Input: part model. Units: mm. Frame: model coordinates. Face numbers are marked on the shaded views. A direction names the side the tool comes from. Coordinates: 2 decimals unless noted, no trailing zeros. Order: outer loops, then holes, each group sorted by start corner. A loop starts at its lowest first (then second) coordinate and runs counter-clockwise, first axis right, second up. Notation, with made-up numbers: (88.25, 11) -> (101.25, 11) arc R28 ccw to (101.25, 33) -> close; hole circle Ø5 at (52.25, 34.25). An arc over 180 degrees is marked (long way). Write each question's results on one line, items separated by ' | '.
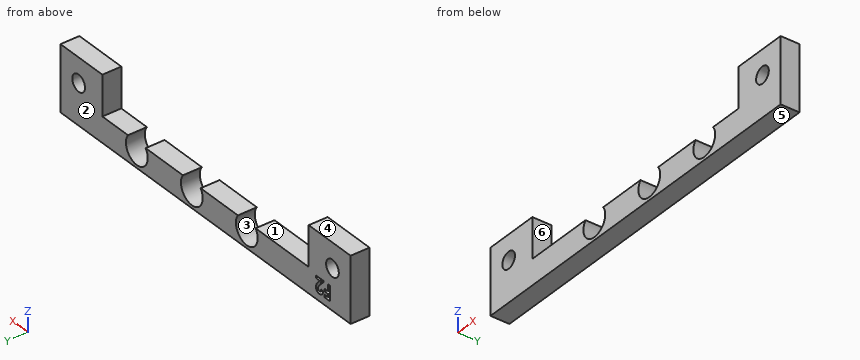
```python
from build123d import *

# Parameters (mm, degrees)
BOSS_EXTRUDE1_OUTLINE_R = 1.75
BOSS_EXTRUDE1_DEPTH     = 4
CUT_EXTRUDE1_DEPTH      = 1


# Read off the part's stored shape, not the designer's step: Boss-Extrude1
with BuildPart() as part:
    # Boss-Extrude1 outline → Boss-Extrude1 (new body)
    with BuildSketch(Plane(origin=(0, 0, 0), x_dir=(1, 0, 0), z_dir=(0, 1, 0))):
        with BuildLine():
            Line((59.039776182, -18.816315938), (59.039776182, -4.977921029))
            Line((59.039776182, -4.977921029), (-20.960223818, -4.977921029))
            Line((-20.960223818, -4.977921029), (-20.960223818, -18.816315938))
            Line((-20.960223818, -18.816315938), (-9.410223818, -18.816315938))
            Line((-9.410223818, -18.816315938), (-9.410223818, -10.337441858))
            Line((-9.410223818, -10.337441858), (5.23307726, -10.337441858))
            ThreePointArc((5.23307726, -10.337441858), (7.669776182, -5.587442326), (10.106475105, -10.337441858))
            Line((10.106475105, -10.337441858), (20.39307726, -10.337441858))
            ThreePointArc((20.39307726, -10.337441858), (22.829776183, -5.587442326), (25.266475105, -10.337441858))
            Line((25.266475105, -10.337441858), (35.55307726, -10.337441858))
            ThreePointArc((35.55307726, -10.337441858), (37.989776182, -5.587442326), (40.426475105, -10.337441858))
            Line((40.426475105, -10.337441858), (47.489776182, -10.337441858))
            Line((47.489776182, -10.337441858), (47.489776182, -18.816315938))
            Line((47.489776182, -18.816315938), (59.039776182, -18.816315938))
        make_face()
        with Locations((-15.960223818, -13.587442209)):
            Circle(BOSS_EXTRUDE1_OUTLINE_R, mode=Mode.SUBTRACT)
        with Locations((54.039776182, -13.587442209)):
            Circle(BOSS_EXTRUDE1_OUTLINE_R, mode=Mode.SUBTRACT)
    extrude(amount=BOSS_EXTRUDE1_DEPTH)

    # Sketch2 → Cut-Extrude1 (cut)
    with BuildSketch(Plane(origin=(0, 4, 0), x_dir=(1, 0, 0), z_dir=(0, 1, 0))):
        Polygon((-15.320752279, -6.539659084), (-13.773957408, -6.539659084), (-13.773957408, -7.109530878), (-14.750880484, -7.109530878), (-14.750880484, -7.720107802), (-13.773957408, -7.720107802), (-13.773957408, -8.289979596), (-14.750880484, -8.289979596), (-14.750880484, -9.714659084), (-15.320752279, -9.714659084), align=None)
        with BuildLine():
            Line((-12.837739459, -7.597992417), (-13.407611254, -7.597992417))
            add(Edge.make_bspline(
                [(-13.407611254, -7.597992417), (-13.405150065, -7.554884631), (-13.40034105, -7.470654604), (-13.381212002, -7.348307794), (-13.355579735, -7.232703511), (-13.321370072, -7.124246154), (-13.278383392, -7.022975131), (-13.227725853, -6.928545205), (-13.16810327, -6.84145355), (-13.100784607, -6.762120173), (-13.026912751, -6.690949467), (-12.948021354, -6.627845049), (-12.862903665, -6.575772871), (-12.773114854, -6.53292229), (-12.678670211, -6.498686666), (-12.57867614, -6.475797382), (-12.473998445, -6.460296534), (-12.402338086, -6.458940148), (-12.365814379, -6.458248827)],
                knots=[0, 0, 0, 0, 1.199038563, 2.342849363, 3.436047546, 4.486744587, 5.497670872, 6.488682221, 7.459191391, 8.424610317, 9.374430501, 10.305433194, 11.225809216, 12.140057399, 13.06607119, 14.010487599, 14.985989317, 16, 16, 16, 16], degree=3))
            add(Edge.make_bspline(
                [(-12.365814379, -6.458248827), (-12.320982046, -6.459647714), (-12.233458825, -6.462378669), (-12.106280643, -6.485674624), (-11.987510127, -6.524640707), (-11.877233611, -6.579086602), (-11.776389898, -6.648254404), (-11.684995712, -6.730725688), (-11.605814958, -6.828230745), (-11.538345606, -6.936712548), (-11.482286639, -7.05157951), (-11.44300285, -7.170356712), (-11.417182038, -7.289892289), (-11.414428089, -7.370381495), (-11.413059972, -7.410367217)],
                knots=[0, 0, 0, 0, 1.075374347, 2.099382735, 3.09057751, 4.06680945, 5.040638231, 6.016817125, 7.011024321, 8.044445721, 9.0776792, 10.070479129, 11.0414456, 12, 12, 12, 12], degree=3))
            add(Edge.make_bspline(
                [(-11.413059972, -7.410367217), (-11.413592644, -7.434553407), (-11.414664782, -7.483234233), (-11.422119502, -7.556900272), (-11.433303054, -7.631937745), (-11.450165124, -7.708282315), (-11.471193509, -7.785955382), (-11.496703979, -7.865189395), (-11.527288275, -7.945535126), (-11.562436007, -8.027896853), (-11.604367341, -8.112541972), (-11.65319055, -8.200739347), (-11.710201514, -8.292410738), (-11.774711612, -8.388073754), (-11.847034153, -8.487577518), (-11.927522194, -8.590622294), (-12.0152487, -8.697571179), (-12.077510669, -8.769060507), (-12.109499275, -8.805789893)],
                knots=[0, 0, 0, 0, 0.728284026, 1.46585585, 2.227944881, 3.01186502, 3.81876927, 4.650621989, 5.517437689, 6.406905708, 7.346299482, 8.360816762, 9.441613733, 10.596154504, 11.834900912, 13.145207542, 14.533280747, 16, 16, 16, 16], degree=3))
            Line((-12.109499275, -8.805789893), (-12.440864459, -9.185492417))
            Line((-12.440864459, -9.185492417), (-11.372354843, -9.185492417))
            Line((-11.372354843, -9.185492417), (-11.372354843, -9.714659084))
            Line((-11.372354843, -9.714659084), (-13.48902151, -9.714659084))
            Line((-13.48902151, -9.714659084), (-13.48902151, -9.42590708))
            Line((-13.48902151, -9.42590708), (-12.548987456, -8.425451351))
            add(Edge.make_bspline(
                [(-12.548987456, -8.425451351), (-12.521771054, -8.396267747), (-12.469060955, -8.33974776), (-12.394059917, -8.256742146), (-12.326190603, -8.1779718), (-12.266860337, -8.102597976), (-12.212955546, -8.033065495), (-12.166879838, -7.96727856), (-12.128211657, -7.905831909), (-12.086231862, -7.83173798), (-12.046364857, -7.743367785), (-12.009784466, -7.641561697), (-11.987486187, -7.544258523), (-11.984408319, -7.480853684), (-11.982931767, -7.450436327)],
                knots=[0, 0, 0, 0, 1.246127091, 2.413378631, 3.493388633, 4.492180848, 5.408488754, 6.240484944, 6.999099869, 7.674939598, 8.898438119, 10.020720584, 11.050475521, 12, 12, 12, 12], degree=3))
            add(Edge.make_bspline(
                [(-11.982931767, -7.450436327), (-11.984035749, -7.421009882), (-11.986174893, -7.363991425), (-12.009682351, -7.282882975), (-12.046100921, -7.209447553), (-12.097419828, -7.145879492), (-12.159583098, -7.093641402), (-12.231418596, -7.054788177), (-12.312340651, -7.032370045), (-12.369068553, -7.029564096), (-12.398251278, -7.028120622)],
                knots=[0, 0, 0, 0, 1.062038974, 2.057870785, 3.028805853, 4.01125022, 4.991535629, 5.949134679, 6.94496649, 8, 8, 8, 8], degree=3))
            add(Edge.make_bspline(
                [(-12.398251278, -7.028120622), (-12.413327445, -7.028653859), (-12.443007301, -7.02970362), (-12.48663437, -7.0366916), (-12.528148661, -7.049007186), (-12.56801225, -7.065508337), (-12.605799703, -7.087380731), (-12.641415708, -7.114341941), (-12.675235525, -7.145706822), (-12.707104042, -7.1813773), (-12.736108553, -7.221185564), (-12.761870254, -7.264768046), (-12.783170892, -7.312097695), (-12.801924747, -7.362549685), (-12.816388618, -7.416665914), (-12.82692011, -7.4741225), (-12.834926501, -7.534825971), (-12.836784749, -7.576553899), (-12.837739459, -7.597992417)],
                knots=[0, 0, 0, 0, 0.903469896, 1.778625579, 2.63899355, 3.493148037, 4.358286772, 5.247621495, 6.164656832, 7.118446693, 8.109501108, 9.111810964, 10.146451449, 11.215617525, 12.33435995, 13.498009769, 14.714554818, 16, 16, 16, 16], degree=3))
        make_face()
    extrude(amount=-CUT_EXTRUDE1_DEPTH, mode=Mode.SUBTRACT)


solid = part.part
```
(1) Cut plane B-B, the plane x = 53. Return loops of the section in (y, z).
Return value:
outline: (0, 4.98) -> (4, 4.98) -> (4, 12.18) -> (0, 12.18) -> close; (0, 15) -> (4, 15) -> (4, 18.82) -> (0, 18.82) -> close
(2) Cut plane A-A, the plane z = 16.25. Return loops of the section in (x, y).
Return value:
outline: (-20.96, 0) -> (-9.41, 0) -> (-9.41, 4) -> (-20.96, 4) -> close; (47.49, 0) -> (59.04, 0) -> (59.04, 4) -> (47.49, 4) -> close
(3) Pin query (flat end, axial travel): P1, Ø2, axis at x = 17, y = 2.5, coming from the +Z side. Return the tip coordinate at first contact, or that it passes through.
Return value:
P1: z = 10.34
(4) Cut plane C-C, the plane y = 1.7. Return loops of the section in (x, z), plus the area to 3 significant figures.
Return value:
outline: (-20.96, 4.98) -> (59.04, 4.98) -> (59.04, 18.82) -> (47.49, 18.82) -> (47.49, 10.34) -> (40.43, 10.34) arc R3 cw (long way) to (35.55, 10.34) -> (25.27, 10.34) arc R3 cw (long way) to (20.39, 10.34) -> (10.11, 10.34) arc R3 cw (long way) to (5.23, 10.34) -> (-9.41, 10.34) -> (-9.41, 18.82) -> (-20.96, 18.82) -> close; hole circle Ø3.5 at (-15.96, 13.59); hole circle Ø3.5 at (54.04, 13.59) | area: 533 mm2
(5) Mould query, pull axis Z, two halves, no side actions, for the marked faces 3, 4, 5 and 6. Classes: +Z half, -Z half, draft (parallel to the pull), parting line (faces both ways), or undercut.
Return value:
face 3: undercut | face 4: +Z half | face 5: -Z half | face 6: draft
(6) Line query: line 1 along X through (y, z) = (2.8, 13.5); line 2 along X through (y, z) = (2.1, 17); line 3 along X through (y, z) = (3.55, 14.75). Output: solid intervals per line, ascending. Write a range as from..to.
Return value:
line 1: -20.96..-17.71, -14.21..-9.41, 47.49..52.29, 55.79..59.04 | line 2: -20.96..-9.41, 47.49..59.04 | line 3: -20.96..-17.27, -14.65..-9.41, 47.49..52.73, 55.35..59.04
(7) Cut plane D-D, the plane x = 38.5. Return loops of the section in (y, z).
Return value:
outline: (0, 4.98) -> (4, 4.98) -> (4, 5.63) -> (0, 5.63) -> close
(8) Reachability of the marked faces 1 and 2 from +Z, -Z, +X, -X, +Y, -Y: full face, straight path, thin tool, end or side. Return the list, or none.
Return value:
face 1: +Z, +Y, -Y | face 2: +Z, -Z, +X, -X, +Y
